Autodesk Inventor part; units mm, degrees
ref_plane "YZ Plane" through (0, 0, 0) normal (1, 0, 0) x (0, 1, 0)
ref_plane "XZ Plane" through (0, 0, 0) normal (0, 1, 0) x (-1, 0, 0)
ref_plane "XY Plane" through (0, 0, 0) normal (0, 0, 1) x (1, 0, 0)
sketch "Sketch1" plane through (0, 0, 0) normal (0, 1, 0) x (-1, 0, 0)
  line L0 (0, 0) -> (25.4, 0)
  line L1 (25.4, 0) -> (25.4, -25.4)
  line L2 (25.4, -50.8) -> (0, -50.8)
  line L3 (0, -50.8) -> (0, 0)
  line L4 (25.4, -50.8) -> (50.8, -50.8)
  line L5 (50.8, -50.8) -> (50.8, -25.4)
  line L6 (50.8, -25.4) -> (25.4, -25.4)
  line L7 (12.7, 0) -> (12.7, -12.7) construction
  line L8 (12.7, -12.7) -> (12.7, -25.4) construction
  line L9 (12.7, -25.4) -> (12.7, -38.1) construction
  line L10 (12.7, -38.1) -> (25.4, -38.1) construction
  line L11 (25.4, -38.1) -> (38.1, -38.1) construction
  line L12 (38.1, -38.1) -> (50.8, -38.1) construction
  circle A0 centre (12.7, -12.7) radius 2.5797
  circle A1 centre (12.7, -25.4) radius 2.5797
  circle A2 centre (12.7, -38.1) radius 2.5797
  circle A3 centre (25.4, -38.1) radius 2.5797
  circle A4 centre (38.1, -38.1) radius 2.5797
  dimension "d0" = 25.4
  dimension "d2" = 25.4
  dimension "d3" = 25.4
  dimension "d4" = 12.7
  dimension "d5" = 12.7
  dimension "d6" = 12.7
  dimension "d7" = 5.1594
  dimension "d8" = 5.1594
  dimension "d9" = 5.1594
  dimension "d10" = 5.1594
  dimension "d11" = 5.1594
extrude "Extrusion1" add sketch "Sketch1" along normal blind 3.175
properties part number "8020 connector"
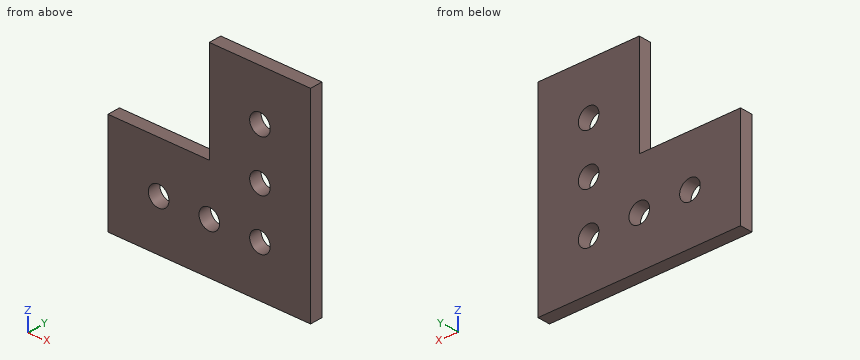
Read the model definition and answer for the solid it produces. Units are mm, in the model's axes. Round coordinates to 2 decimals unless told otherwise and drop trailing zeros. Write each loop counter-clockwise with the first axis right and the second up, starting at its lowest first coordinate (ties: lowest second). Pieces come first, ordered by that corner, then holes.
Q1. Straight lines are drawn through the part: line 1 (Z direction, x = -12.7, y = 1.35); line 2 (Z direction, x = -11, y = 2.9); line 3 (Z direction, x = -38.1, y = 1.35). For each, find the intervals that lie inside material, in ascending order.
Values:
line 1: z = -50.8 to -40.68, -35.52 to -27.98, -22.82 to -15.28, -10.12 to 0
line 2: z = -50.8 to -40.04, -36.16 to -27.34, -23.46 to -14.64, -10.76 to 0
line 3: z = -50.8 to -40.68, -35.52 to -25.4
Q2. Find section D-D on y = 0.9. Determine the outline of the cut face in (x, z), and give its area (3 significant figures).
Values:
outline: (-50.8, -50.8) - (0, -50.8) - (0, 0) - (-25.4, 0) - (-25.4, -25.4) - (-50.8, -25.4) - close; hole circle Ø5.16 at (-38.1, -38.1); hole circle Ø5.16 at (-25.4, -38.1); hole circle Ø5.16 at (-12.7, -38.1); hole circle Ø5.16 at (-12.7, -25.4); hole circle Ø5.16 at (-12.7, -12.7)
area: 1,830 mm2
Q3. Find section B-B on x = -12.7. Determine the outline of the cut face in (y, z) (3 decimals).
Values:
outline: (0, -50.8) - (3.175, -50.8) - (3.175, -40.68) - (0, -40.68) - close; (0, -35.52) - (3.175, -35.52) - (3.175, -27.98) - (0, -27.98) - close; (0, -22.82) - (3.175, -22.82) - (3.175, -15.28) - (0, -15.28) - close; (0, -10.12) - (3.175, -10.12) - (3.175, 0) - (0, 0) - close
Q4. Find section C-C on z = -12.7. Determine the outline of the cut face in (x, y) (3 decimals).
Values:
outline: (-25.4, 0) - (-15.28, 0) - (-15.28, 3.175) - (-25.4, 3.175) - close; (-10.12, 0) - (0, 0) - (0, 3.175) - (-10.12, 3.175) - close
Q5. Find section A-A on x = -38.1. Determine the outline of the cut face in (y, z) (3 decimals).
Values:
outline: (0, -50.8) - (3.175, -50.8) - (3.175, -40.68) - (0, -40.68) - close; (0, -35.52) - (3.175, -35.52) - (3.175, -25.4) - (0, -25.4) - close
Q6. Flat-ended cylindrical pins translate along their axes: P1, Ø1, axis at x = -19.5, z = -37.5, coming from the -Y side; P2, Ø1.6, axis at y = 2, z = -7.5, coming from the -X side; P3, Ø1, axis at x = -38, y = 2, coming from the +Z side. Find the tip coordinate at first contact, or state that the pin passes through.
Values:
P1: stops at y = 0
P2: stops at x = -25.4
P3: stops at z = -25.4
